```python
from build123d import *

# Parameters (mm, degrees)
SKETCH1_R               = 3.35
BOSS_EXTRUDE1_DEPTH     = 9
SKETCH2_R               = 3.9
BOSS_EXTRUDE2_DEPTH     = 30
CHAMFER1_SIZE           = 1
CHAMFER2_SIZE           = 1
CUT_EXTRUDE1_DEPTH      = 40.38806926
CUT_EXTRUDE1_DEPTH_BACK = 40.38806926
SKETCH8_R               = 2


with BuildPart() as part:
    # Sketch1 → Boss-Extrude1 (new body)
    with BuildSketch(Plane(origin=(0, 0, 0), x_dir=(0, 1, 0), z_dir=(0, 0, 1))):
        with Locations(Location((0, 0, 0), (0, 0, 270))):
            Circle(SKETCH1_R)
    extrude(amount=BOSS_EXTRUDE1_DEPTH)

    # Sketch2 → Boss-Extrude2 (add)
    with BuildSketch(Plane.XY.offset(9)):
        Circle(SKETCH2_R)
    extrude(amount=BOSS_EXTRUDE2_DEPTH)

    # Chamfer1
    # the kernel refuses this chamfer: 1 mm, written as the material it adds along each edge
    with BuildSketch(Plane(origin=(0, 0, 9), x_dir=(1, 0, 0), z_dir=(0, -1, 0))) as chamfer1_piece_1_section:
        Polygon((3.35 + CHAMFER1_SIZE, 0), (3.35, -CHAMFER1_SIZE), (3.35, 0), align=None)
    chamfer1_piece_1 = revolve(axis=Axis((0, 0, 9), (0, 0, 1)), mode=Mode.PRIVATE)
    chamfer1_piece_1 = chamfer1_piece_1 & Plane(origin=(0, 0, 8.27596247), x_dir=(1, 0, 0), z_dir=(0, 0, -1)) * Cylinder(3.9, 18, mode=Mode.PRIVATE)
    add(chamfer1_piece_1)

    # Chamfer2
    chamfer2_edges = [part.edges().sort_by_distance(p)[0] for p in [
        (-3.35, 0, 0),
    ]]
    chamfer(chamfer2_edges, length=CHAMFER2_SIZE)

    # Sketch8 → Cut-Extrude1 (cut, two sides: drawn at the far end of the back side and taken through both)
    with BuildSketch(Plane.XY.offset(39).offset(-CUT_EXTRUDE1_DEPTH_BACK)):
        Circle(SKETCH8_R)
    extrude(amount=CUT_EXTRUDE1_DEPTH + CUT_EXTRUDE1_DEPTH_BACK, mode=Mode.SUBTRACT)


solid = part.part
```
Design review of the part built by this model. Coordinates are the model's own, in mm. Coordinates: 2 decimals unless noted, no trailing zeros. Loops run counter-clockwise (first coordinate to the right, second up) from the corner with the lowest first, then second, coordinate; pieces in that order, holes last.
Q1. We need section A-A on x = 0. State the section outline as (y, z) points, and give its area (3 significant figures).
Reported:
outline: (-3.9, 8.55) - (-3.35, 8) - (-3.35, 1) - (-2.35, 0) - (-2, 0) - (-2, 39) - (-3.9, 39) - close; (2, 0) - (2.35, 0) - (3.35, 1) - (3.35, 8) - (3.9, 8.55) - (3.9, 39) - (2, 39) - close
area: 138 mm2
Q2. To check wall thickness, follow line 1 (Y direction, x = 0, z = 9); line 2 (Y direction, x = 0.5, z = 8.5). State the ranges of each line that lie inside material, in increasing order.
Reported:
line 1: y = -3.9 to -2, 2 to 3.9
line 2: y = -3.82 to -1.94, 1.94 to 3.82
Q3. We need section C-C on z = 4.5. State the section outline as (x, y) points, and give its area (3 significant figures).
Reported:
outline: circle Ø6.7 at (0, 0); hole circle Ø4 at (0, 0)
area: 22.7 mm2
Q4. We need section D-D on z = 25. State the section outline as (x, y) points, and give its area (3 significant figures).
Reported:
outline: circle Ø7.8 at (0, 0); hole circle Ø4 at (0, 0)
area: 35.2 mm2
Q5. The part is to be moulded in two halves that separate along Y. For faces 1 (the face through (0, -2, 19)), 2 (the face through (-2, 1, 39)), 3 (the face through (-2.87, -2.64, 23.56)), say which applies: +Y half, -Y half, draft (parallel to the pull), parting line (faces both ways), or undercut.
Reported:
face 1: undercut
face 2: draft
face 3: parting line
